Verification items for the finished model (mm, model axes). Face numbers are marked on the shaded views. A direction names the side the tool comes from. Give positions to 0.01 mm unless a question says otherwise; leave off trailing zeros. Loops run counter-clockwise (first coordinate to the right, second up) from the corner with the lowest first, then second, coordinate; pieces in that order, holes last. Notation, with made-up numbers: (40, 71) - (58, 71) arc R20 cw to (58, 89) - close; hole circle Ø3 at (65, 75). An arc over 180 degrees is marked (long way). One line per item, written item: value. Start each with the question number.
1. Sectioned sample at B-B (x = -12.5). Record the cut outline in (y, z).
2. Sectioned sample at D-D (y = -45). Record the cut outline in (x, z).
3. Sectioned sample at A-A (y = -13). Record the cut outline in (x, z).
4. Gauge pin test, flat ends, axial feed: pin 1 (2.5 mm diameter, centred on y = -51, z = 1.5, fed in from +X); pin 2 (10.5 mm diameter, centred on x = -15.35, y = -7.18, fed in from +Z); pin 3 (6 mm diameter, centred on x = -0.5, y = -7.5, fed in from -Z); pin 4 (2.5 mm diameter, centred on x = 21.5, z = 1.5, fed in from -Y). Record the tip position at first contact, or that the pin passes through.
5. Scan lines: L1, parallel to X at y = -3, z = 3.2; L2, parallel to X at y = -8, z = 4.6; L3, parallel to Y at x = -11, z = 3.65. Record each from-to range of solid material in increasing order. Write a range as [from, to].
6. Sectioned sample at C-C (z = 4.3). Count the separate pieces of the cut face and the enclosed holes in it, plus the area to 3 significant figures.
7. Access from +Z, -Z, +X, -X, +Y, -Y to the whole of each face (thin tool, end or side, straight path). Record for the marked faces 5 and 6.
8. Mould release check, pull along Y, two halves, no side actions. Record for the marked faces 1, 2, 3 and 4: pulls with the +Y half, pulls with the -Y half, needs draft (parallel to the pull), parting line crosses it, or undercut.
from build123d import *

# Parameters (mm, degrees)
SKETCH2_R           = 6.45
BOSS_EXTRUDE1_DEPTH = 5
CUT_EXTRUDE1_START  = -57.18341
SKETCH3_W           = 3.1
SKETCH3_H           = 5
CUT_EXTRUDE1_DEPTH  = 15
FILLET1_R           = 5


with BuildPart() as part:
    # Sketch2 → Boss-Extrude1 (new body)
    with BuildSketch(Plane.XY):
        with BuildLine():
            Line((22.650655022, -27.183406114), (22.650655022, -57.183406114))
            ThreePointArc((22.650655022, -57.183406114), (-9.462495777, -37.680698146), (-25.349344978, -3.633406114))
            Line((-25.349344978, -3.633406114), (-25.349344978, 2.816593886))
            Line((-25.349344978, 2.816593886), (19.650655022, 2.816593886))
            Line((19.650655022, 2.816593886), (19.650655022, -2.183406114))
            ThreePointArc((19.650655022, -2.183406114), (20.403335755, -14.773084426), (22.650655022, -27.183406114))
        make_face()
        with Locations((9.650655022, -7.183406114)):
            Circle(SKETCH2_R, mode=Mode.SUBTRACT)
        with Locations((-15.349344978, -7.183406114)):
            Circle(SKETCH2_R, mode=Mode.SUBTRACT)
    extrude(amount=BOSS_EXTRUDE1_DEPTH)

    # Sketch3 → Cut-Extrude1 (cut)
    with BuildSketch(Plane(origin=(0, 0, 0), x_dir=(1, 0, 0), z_dir=(0, 1, 0)).offset(CUT_EXTRUDE1_START)):
        with Locations((21.100655022, -2.5)):
            Rectangle(SKETCH3_W, SKETCH3_H)
    extrude(amount=CUT_EXTRUDE1_DEPTH, mode=Mode.SUBTRACT)

    # Fillet1
    fillet1_edges = [part.edges().sort_by_distance(p)[0] for p in [
        (-25.349344978, 2.816593886, 2.5),
        (19.650655022, 2.816593886, 2.5),
    ]]
    fillet(fillet1_edges, radius=FILLET1_R - 0.0001)  # a hair under: the kernel refuses the full size


solid = part.part
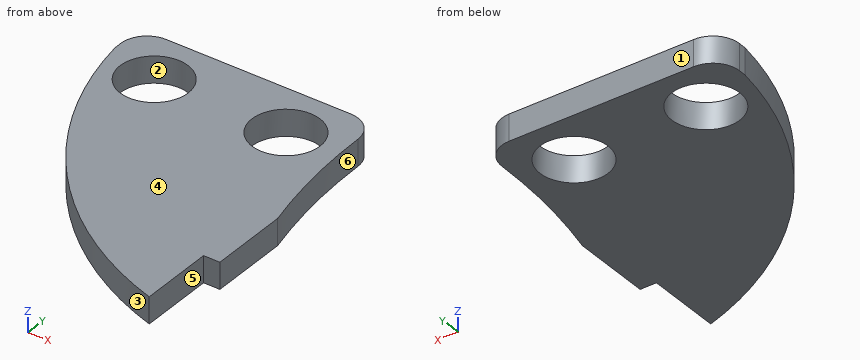
Results are:
1. outline: (-34.03, 0) - (-12.97, 0) - (-12.97, 5) - (-34.03, 5) - close; (-1.4, 0) - (2.82, 0) - (2.82, 5) - (-1.4, 5) - close
2. outline: (-1.73, 0) - (19.55, 0) - (19.55, 5) - (-1.73, 5) - close
3. outline: (-23.29, 0) - (-18.14, 0) - (-18.14, 5) - (-23.29, 5) - close; (-12.56, 0) - (6.86, 0) - (6.86, 5) - (-12.56, 5) - close; (12.44, 0) - (20.21, 0) - (20.21, 5) - (12.44, 5) - close
4. pin 1: stops at x = 19.55
4. pin 2: passes through
4. pin 3: stops at z = 0
4. pin 4: stops at y = -42.18
5. L1: x = [-25.35, -20.26], [-10.44, 4.74], [14.56, 19.65]
5. L2: x = [-24.57, -21.75], [-8.95, 3.25], [16.05, 19.81]
5. L3: y = [-35.9, -11.95], [-2.42, 2.82]
6. separate pieces: 1
6. enclosed holes: 2
6. area: 1,740 mm^2
7. face 5: +Z, -Z, +X, -Y
7. face 6: +Z, -Z, +X, +Y
8. face 1: pulls with the +Y half
8. face 2: undercut
8. face 3: pulls with the -Y half
8. face 4: needs draft
